Could you check a few things on this model? Use its own coordinates, in mm. Face numbers are marked on the shaded views. Round coordinates to 2 decimals unless told otherwise and drop trailing zeros. Loops run counter-clockwise (first coordinate to the right, second up) from the corner with the lowest first, then second, coordinate; pieces in that order, holes last. Notation, with made-up numbers: M 79,-19.5 L 83,-19.5 A30 cw 83,10.5 Z; hole C 60,67.25 d3. An arc over 180 degrees is marked long. Return JSON: item names as keys, results as strings. Group by question number.
```python
from build123d import *

# Parameters (mm, degrees)
F0_R     = 36.5
F1_DEPTH = 20
F2_T     = -1.5
F3_R     = 2
F5_DEPTH = 50


with BuildPart() as f1:
    # F0 (on Top) → F1 (new body)
    with BuildSketch(Plane.XY):
        Circle(F0_R)
    extrude(amount=F1_DEPTH)

    # F2
    f2_openings = [f1.faces().sort_by_distance(p)[0] for p in [
        (0, 0, 20),
    ]]
    offset(amount=F2_T, openings=f2_openings)

    # F3
    f3_edges = [f1.edges().sort_by_distance(p)[0] for p in [
        (-36.5, 0, 0),
    ]]
    fillet(f3_edges, radius=F3_R)

    # F4 (on Front) → F5 (cut, symmetric)
    with BuildSketch(Plane.XZ):
        with BuildLine():
            Line((-2.5, 11), (-2.5, 9.5))
            ThreePointArc((-2.5, 9.5), (0, 7), (2.5, 9.5))
            Line((2.5, 9.5), (2.5, 11))
            ThreePointArc((2.5, 11), (0, 13.5), (-2.5, 11))
        make_face()
    extrude(amount=F5_DEPTH, both=True, mode=Mode.SUBTRACT)


solid = f1.part
```
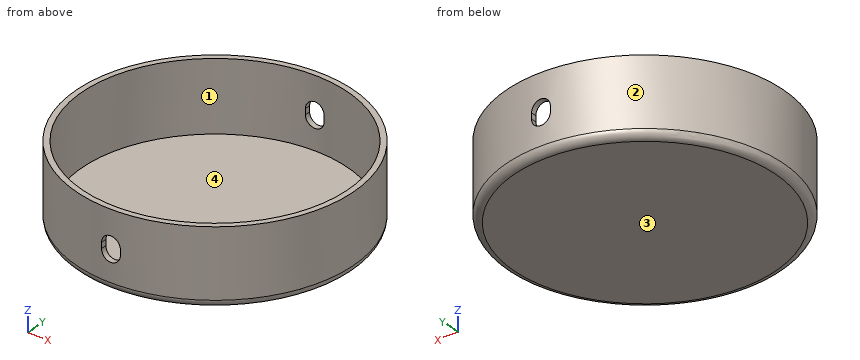
1. I need wall thicknesses on probe 1 along Y at (x, z) = (0, 5.5); probe 2 along X at (y, z) = (-1, 2.5); probe 3 along Z at (x, y) = (12, 13). Which ranges of each line are inside material? Lowest first, please.
2. If we section it at D-D, the plane z = 14.5: Please give me the cut outline in (x, y).
3. I'm going to push flat-ended pins straight in: pin 1 Ø1.5 at (x, z) = (11.5, 5) entering from +Y; pin 2 Ø1 at (y, z) = (-5.5, 10.5) entering from -X; pin 3 Ø1.5 at (y, z) = (2, 10) entering from +X. Where does each tip first touch, or does it pass through?
4. We'd pull the mould along Y, two halves only. Please class the marked faces 1, 2, 3 and 4: +Y half, -Y half, draft (parallel to the pull), parting line (faces both ways), or undercut.
5. If we section it at C-C, the plane y = 0: Please give me the cut outline in (x, z), then the cut area to 3 significant figures.
6. If we section it at A-A, the plane x = 0: Please give me the cut outline in (y, z).
Geometry results:
{
 "1": {"probe 1": "-36.5 to -35, 35 to 36.5", "probe 2": "-36.49 to -34.99, 34.99 to 36.49", "probe 3": "0 to 1.5"},
 "2": {"outline": "C 0,0 d73; hole C 0,0 d70"},
 "3": {"pin 1": "y = 34.88", "pin 2": "x = -36.16", "pin 3": "x = 36.48"},
 "4": {"face 1": "undercut", "face 2": "parting line", "face 3": "draft", "face 4": "undercut"},
 "5": {"outline": "M -36.5,2 A2 ccw -34.5,0 L 34.5,0 A2 ccw 36.5,2 L 36.5,20 L 35,20 L 35,1.5 L -35,1.5 L -35,20 L -36.5,20 Z", "area": "163 mm^2"},
 "6": {"outline": "M -36.5,2 A2 ccw -34.5,0 L 34.5,0 A2 ccw 36.5,2 L 36.5,7 L 35,7 L 35,1.5 L -35,1.5 L -35,7 L -36.5,7 Z; M -36.5,13.5 L -35,13.5 L -35,20 L -36.5,20 Z; M 35,13.5 L 36.5,13.5 L 36.5,20 L 35,20 Z"}
}
